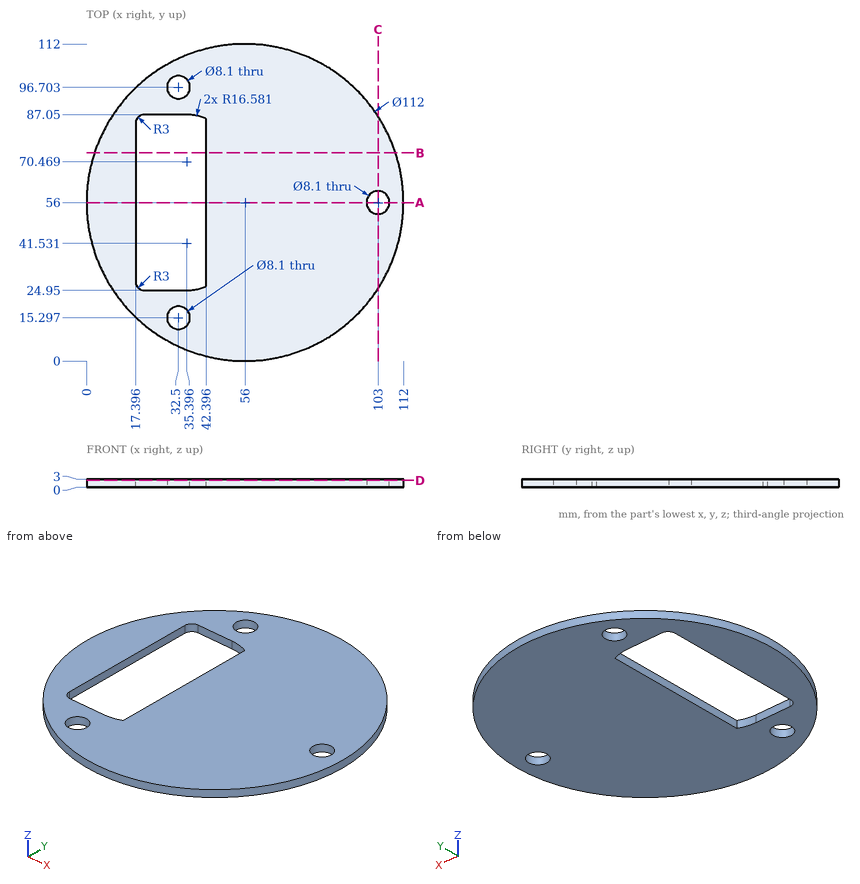
Can you work these out from the drawing? Everything is in mm from the part's minimum corner. Coordinates: 2 decimals unless noted, no trailing zeros. Order: outer loops, then holes, each group sorted by start corner. A loop starts at its lowest first (then second) coordinate and runs counter-clockwise, first axis right, second up. Notation, with made-up numbers: (64, 5.5) -> (110, 5.5) arc R17 cw to (110, 19.5) -> close; hole circle Ø7 at (-4.5, 55). An arc over 180 degrees is marked (long way). Use one line per item in the form item = value.
Q1. Imagine slicing it at C-C, the plane x = 103. List the corners of the cut face in (y, z) for me, then the cut area to 3 significant figures.
From the geometry:
outline = (25.55, 0) -> (51.95, 0) -> (51.95, 3) -> (25.55, 3) -> close; (60.05, 0) -> (86.45, 0) -> (86.45, 3) -> (60.05, 3) -> close
area = 158 mm²
Q2. Imagine slicing it at D-D, the plane z = 2.5. List the corners of the cut face in (x, y) for me, then the cut area to 3 significant figures.
From the geometry:
outline = circle Ø112 at (56, 56); hole (17.4, 27.95) arc R3 ccw to (20.4, 24.95) -> (35.4, 24.95) arc R16.58 ccw to (42.4, 26.5) -> (42.4, 85.5) arc R16.58 ccw to (35.4, 87.05) -> (20.4, 87.05) arc R3 ccw to (17.4, 84.05) -> close; hole circle Ø8.1 at (32.5, 15.3); hole circle Ø8.1 at (32.5, 96.7); hole circle Ø8.1 at (103, 56)
area = 8,160 mm²
Q3. I need wall thicknesses on L1, parallel to Y at x = 32.5, z = 1.85; L2, parallel to Y at x = 55.5, z = 1.7; L3, parallel to X at y = 50.5, z = 1.65. Which ranges of each line are inside material? Lowest first, please.
From the geometry:
L1 = 5.17 to 11.25, 19.35 to 24.95, 87.05 to 92.65, 100.75 to 106.83
L2 = 0 to 112
L3 = 0.27 to 17.4, 42.4 to 111.73
Q4. Imagine slicing it at A-A, the plane y = 56. List the corners of the cut face in (x, z) for me.
From the geometry:
outline = (0, 0) -> (17.4, 0) -> (17.4, 3) -> (0, 3) -> close; (42.4, 0) -> (98.95, 0) -> (98.95, 3) -> (42.4, 3) -> close; (107.05, 0) -> (112, 0) -> (112, 3) -> (107.05, 3) -> close
Q5. Will these pins go through, and if not, where does the flat tip stop? P1, Ø1.5, axis at y = 59, z = 1, coming from the -X side (1 decimal); P2, Ø1.5, axis at x = 24.5, z = 1.5, coming from the -Y side; P3, Ø1, axis at x = 22, z = 0.5, coming from the -Y side (1 decimal).
From the geometry:
P1 = 0
P2 = 9.2
P3 = 11.1
Q6. Imagine slicing it at B-B, the plane y = 73.5. List the corners of the cut face in (x, z) for me (1 decimal).
From the geometry:
outline = (2.8, 0) -> (17.4, 0) -> (17.4, 3) -> (2.8, 3) -> close; (42.4, 0) -> (109.2, 0) -> (109.2, 3) -> (42.4, 3) -> close
